from build123d import *

# Parameters (mm, degrees)
SKETCH1_R           = 10
BOSS_EXTRUDE1_DEPTH = 2.2
SKETCH2_R           = 1.5
CUT_EXTRUDE1_DEPTH  = 15.31223253
SKETCH2_3_R         = 3.815
BOSS_EXTRUDE2_DEPTH = 9
CHAMFER1_SIZE       = 0.2


with BuildPart() as part:
    # Sketch1 → Boss-Extrude1 (new body)
    with BuildSketch(Plane.XY):
        Circle(SKETCH1_R)
    extrude(amount=BOSS_EXTRUDE1_DEPTH)

    # Sketch2 → Cut-Extrude1 (cut, through all)
    with BuildSketch(Plane.XY.offset(2.2)):
        with Locations((0, 7.7)):
            Circle(SKETCH2_R)
        with Locations((7.7, 0)):
            Circle(SKETCH2_R)
        with Locations((0, -7.7)):
            Circle(SKETCH2_R)
        with Locations((-7.7, 0)):
            Circle(SKETCH2_R)
    extrude(amount=-CUT_EXTRUDE1_DEPTH, mode=Mode.SUBTRACT)

    # Sketch2<3> → Boss-Extrude2 (add)
    with BuildSketch(Plane.XY.offset(2.2)):
        Circle(SKETCH2_3_R)
    extrude(amount=BOSS_EXTRUDE2_DEPTH)

    # Chamfer1
    chamfer1_edges = [part.edges().sort_by_distance(p)[0] for p in [
        (-10, 0, 0),
        (-3.815, 0, 11.2),
        (-10, 0, 2.2),
    ]]
    chamfer(chamfer1_edges, length=CHAMFER1_SIZE)


solid = part.part
The listing builds one solid part. Answer for the finished solid, in the listing's coordinates (mm). A direction names the side the tool comes from. Give positions to 0.01 mm unless a question says otherwise; leave off trailing zeros. Order: outer loops, then holes, each group sorted by start corner. A loop starts at its lowest first (then second) coordinate and runs counter-clockwise, first axis right, second up. Notation, with made-up numbers: (-11, 63.5) - (43, 63.5) arc R26 ccw to (43, 98.5) - close; hole circle Ø3 at (-1, 35). An arc over 180 degrees is marked (long way). Use one line per item in the form item = value.
1) Find section A-A on x = 0. Determine the outline of the cut face in (y, z) (3 decimals).
Verdict:
outline = (-10, 0.2) - (-9.8, 0) - (-9.2, 0) - (-9.2, 2.2) - (-9.8, 2.2) - (-10, 2) - close; (-6.2, 0) - (6.2, 0) - (6.2, 2.2) - (3.815, 2.2) - (3.815, 11) - (3.615, 11.2) - (-3.615, 11.2) - (-3.815, 11) - (-3.815, 2.2) - (-6.2, 2.2) - close; (9.2, 0) - (9.8, 0) - (10, 0.2) - (10, 2) - (9.8, 2.2) - (9.2, 2.2) - close
2) Find section C-C on z = 4.5. Determine the outline of the cut face in (x, y) (3 decimals).
Verdict:
outline = circle Ø7.63 at (0, 0)
3) Consider probe 1 along Y at (x, z) = (0, 1); probe 2 along Z at (x, y) = (-8.25, 3.5); probe 3 along Y at (x, z) = (0.5, 1.75). Determine where each line is inside the solid, lowest interval first. Write a range as [from, to].
Verdict:
probe_1 = [-10, -9.2], [-6.2, 6.2], [9.2, 10]
probe_2 = [0, 2.2]
probe_3 = [-9.99, -9.11], [-6.29, 6.29], [9.11, 9.99]
4) The mould has two halves that part along Y. Classify faces 3 (the cylindrical face through (-0.325, 6.236, 1.115)), 4 (the cylindrical face through (-2.17, -9.76, 1.09)), 5 (the flat face through (0, 0, 11.2)), 6 (the cylindrical face through (-0.195, -6.213, 1.115)): released by +Y, released by -Y, zero draft, split by the parting line, or undercut.
Verdict:
face_3 = undercut
face_4 = split by the parting line
face_5 = zero draft
face_6 = undercut
5) Each of these flat-tipped pins is pushed along its axis until it touches: pin 1 (2.5 mm diameter, centred on x = 0, y = 7.7, fed in from +Z); pin 2 (3 mm diameter, centred on x = 3, y = 7.5, fed in from -Z); pin 3 (5 mm diameter, centred on y = -5.5, z = 6.5, fed in from +X); pin 4 (6 mm diameter, centred on x = -6.5, z = 6, fed in from -Y). Where does it stop, or does it pass through?
Verdict:
pin_1 = through
pin_2 = 0
pin_3 = 2.36
pin_4 = -1.52
6) For faces 1 (the cylindrical face through (6.2, 0.07, 1.12)), 2 (the flat face through (4, 0, 2.2)), determine the directions among +Z, -Z, +X, -X, +Y, -Y from which every point of the face is accessible in a straight line to the end or side of a thin tool.
Verdict:
face_1 = +Z, -Z
face_2 = +Z
